```python
from build123d import *

# Parameters (mm, degrees)
BASE_DEPTH      = 3
SKETCH2_W       = 3
SKETCH2_H       = 5
SKETCH2_R       = 0.509076859
POLARITY_DEPTH  = 0.1
SKETCH3_W       = 0.671157402
SKETCH3_H       = 0.5
SKETCH3_W_2     = 0.596513076
LIGHTSLOT_DEPTH = 6
SKETCH4_W       = 0.3
SKETCH4_H       = 0.4


with BuildPart() as part:
    # Sketch1 → Base (new, symmetric)
    with BuildSketch(Plane.XY):
        Polygon((6.5, 0), (-6.5, 0), (-6.5, 10), (-2.5, 10), (-2.5, 2), (2.5, 2), (2.5, 10), (6.5, 10), align=None)
    extrude(amount=BASE_DEPTH, both=True)

    # Sketch2 → Polarity (cut)
    # profile 1 of 2: a face of its own
    with BuildSketch(Plane(origin=(0, 10, 0), x_dir=(1, 0, 0), z_dir=(0, 1, 0))):
        with Locations((-4.5, 0)):
            Rectangle(SKETCH2_W, SKETCH2_H)
        Polygon((-4.644390506, 1.198307086), (-5.614083966, 1.198307086), (-4.644390506, -0.88812109), (-5.614083966, -0.88812109), (-5.614083966, -1.176902103), (-4.644390506, -1.176902103), (-4.644390506, -1.773829525), (-4.355609494, -1.773829525), (-4.355609494, -1.176902103), (-3.385916034, -1.176902103), (-3.385916034, -0.88812109), (-4.355609494, -0.88812109), (-3.385916034, 1.198307086), (-4.355609494, 1.198307086), (-4.355609494, 1.796472229), (-4.644390506, 1.796472229), align=None, mode=Mode.SUBTRACT)
    # profile 2 of 2: a face of its own
    with BuildSketch(Plane(origin=(0, 10, 0), x_dir=(1, 0, 0), z_dir=(0, 1, 0))):
        with Locations((4.5, 0)):
            Rectangle(SKETCH2_W, SKETCH2_H)
        with Locations(Location((4.492051803, -1.006853172, 0), (0, 0, 180))):
            Circle(SKETCH2_R, mode=Mode.SUBTRACT)
    extrude(amount=-POLARITY_DEPTH, mode=Mode.SUBTRACT)

    # Sketch3 → LightSlot (cut)
    with BuildSketch(Plane(origin=(0, 2, 0), x_dir=(1, 0, 0), z_dir=(0, 1, 0))):
        with Locations((-2.5, 0)):
            Rectangle(SKETCH3_W, SKETCH3_H)
        with Locations((2.5, 0)):
            Rectangle(SKETCH3_W_2, SKETCH3_H)
    extrude(amount=LIGHTSLOT_DEPTH, mode=Mode.SUBTRACT)

    # Sweep1: sweep along a curve in space
    with BuildLine() as sweep1_path:
        Line((5, 0, 1.25), (5, -1.034487075, 1.25))
        ThreePointArc((5, -1.034487075, 1.25), (5.146446609, -1.388040466, 1.25), (5.5, -1.534487075, 1.25))
        Line((5.5, -1.534487075, 1.25), (6.5, -1.534487075, 1.25))
    # Sketch4 → Sweep1 (sweep)
    with BuildSketch(Plane.XZ):
        with Locations((5, 1.25)):
            Rectangle(SKETCH4_W, SKETCH4_H)
        with Locations((5, -1.25)):
            Rectangle(SKETCH4_W, SKETCH4_H)
    sweep1 = sweep(path=sweep1_path.line)

    # Mirror1: Sweep1 across plane
    add(sweep1.mirror(Plane(origin=(0, 0, 0), x_dir=(0, 0, 1), z_dir=(1, 0, 0))))


solid = part.part
```
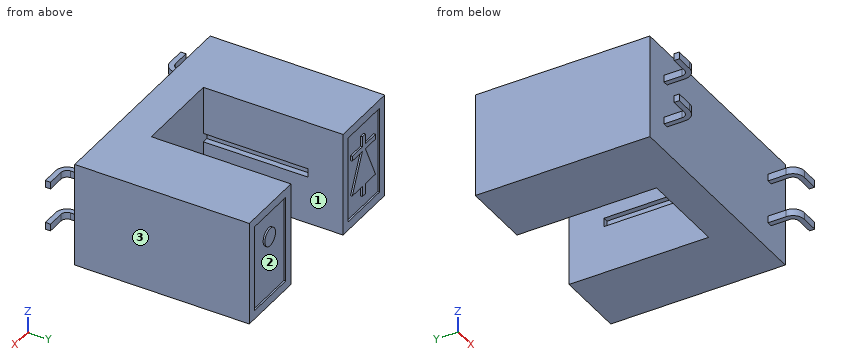
The listing builds one solid part. Answer for the finished solid, in the listing's coordinates (mm). Face numbers are marked on the shaded views. A direction names the side the tool comes from. Coordinates: 2 decimals unless noted, no trailing zeros. Loops run counter-clockwise (first coordinate to the right, second up) from the corner with the lowest first, then second, coordinate; pieces in that order, holes last. Notation, with made-up numbers: (26.25, 65.25) -> (31.25, 65.25) arc R6 ccw to (31.25, 73.25) -> close; hole circle Ø1 at (21, -5.75). An arc over 180 degrees is marked (long way). Use one line per item in the form item = value. Start each with the question number.
Item 1: A tool of negligible diameter and unlimited length cuts with its end or side. For the marked faces 1, 2 and 3, from which of +Z, -Z, +X, -X, +Y, -Y can it reach the whole face along a straight path? Write none if from no direction.
Item 2: The part is cut by section D-D on x = 4.25. Determine the outline of the cut face in (y, z).
Item 3: The part is cut by section C-C on z = 2.05. Determine the outline of the cut face in (x, y), then the cut area to 3 significant figures.
Item 4: Flat-ended cylindrical pins translate along their axes: pin 1 Ø1.8 at (x, y) = (5.5, -0.5) entering from +Z; pin 2 Ø1 at (x, z) = (-3.5, 2.5) entering from -Y. Find the tip coordinate at first contact, or state that the pin passes through.
Item 5: The part is cut by section B-B on y = 2.5. Determine the outline of the cut face in (x, z), then the cut area to 3 significant figures.
Item 6: The part is cut by section A-A on y = -0.5. Determine the outline of the cut face in (x, z).
Item 7: Consider L1, parallel to X at y = 6, z = 1.2; L2, parallel to X at y = 3.25, z = 0.05; L3, parallel to Y at x = 4.5, z = -0.6. Determine where each line is inside the solid, lowest interval first. Write a range as [from, to].
Answer key:
q1.face_1 = +Z, -Z, +Y
q1.face_2 = +Y
q1.face_3 = +Z, -Z, +X, +Y, -Y
q2.outline = (0, -3) -> (10, -3) -> (10, -2.5) -> (9.9, -2.5) -> (9.9, 0.56) -> (10, 0.56) -> (10, 1.45) -> (9.9, 1.45) -> (9.9, 2.5) -> (10, 2.5) -> (10, 3) -> (0, 3) -> close
q3.outline = (-6.5, 0) -> (6.5, 0) -> (6.5, 10) -> (6, 10) -> (6, 9.9) -> (3, 9.9) -> (3, 10) -> (2.5, 10) -> (2.5, 2) -> (-2.5, 2) -> (-2.5, 10) -> (-3, 10) -> (-3, 9.9) -> (-6, 9.9) -> (-6, 10) -> (-6.5, 10) -> close
q3.area = 89.4 mm2
q4.pin_1 = 3
q4.pin_2 = 0
q5.outline = (-6.5, -3) -> (-2.5, -3) -> (-2.5, -0.25) -> (-2.84, -0.25) -> (-2.84, 0.25) -> (-2.5, 0.25) -> (-2.5, 3) -> (-6.5, 3) -> close; (2.5, -3) -> (6.5, -3) -> (6.5, 3) -> (2.5, 3) -> (2.5, 0.25) -> (2.8, 0.25) -> (2.8, -0.25) -> (2.5, -0.25) -> close
q5.area = 47.7 mm2
q6.outline = (-5.15, -1.45) -> (-4.85, -1.45) -> (-4.85, -1.05) -> (-5.15, -1.05) -> close; (-5.15, 1.05) -> (-4.85, 1.05) -> (-4.85, 1.45) -> (-5.15, 1.45) -> close; (4.85, -1.45) -> (5.15, -1.45) -> (5.15, -1.05) -> (4.85, -1.05) -> close; (4.85, 1.05) -> (5.15, 1.05) -> (5.15, 1.45) -> (4.85, 1.45) -> close
q7.L1 = [-6.5, -2.5], [2.5, 6.5]
q7.L2 = [-6.5, -2.84], [2.8, 6.5]
q7.L3 = [0, 9.9]
